from build123d import *


with BuildPart() as part:
    # Sketch1 → Base-Revolve (revolve)
    with BuildSketch(Plane.XY):
        with BuildLine():
            Line((132, 30), (0, 30))
            Line((0, 30), (-132, 30))
            Line((-132, 30), (-132, 28.5))
            Line((-132, 28.5), (-134.15, 28.5))
            Line((-134.15, 28.5), (-134.15, 30))
            Line((-134.15, 30), (-136.323673019, 30))
            ThreePointArc((-136.323673019, 30), (-136.497321197, 29.984807753), (-136.665693163, 29.939692621))
            Line((-136.665693163, 29.939692621), (-137.842020143, 29.511544614))
            ThreePointArc((-137.842020143, 29.511544614), (-138.319152044, 29.14542843), (-138.5, 28.571851993))
            Line((-138.5, 28.571851993), (-138.5, 0))
            Line((-138.5, 0), (115.555513627, 0))
            Line((115.555513627, 0), (118.5, 5.1))
            Line((118.5, 5.1), (138.5, 5.1))
            Line((138.5, 5.1), (138.5, 28.571851993))
            ThreePointArc((138.5, 28.571851993), (138.319152044, 29.14542843), (137.842020143, 29.511544614))
            Line((137.842020143, 29.511544614), (136.665693163, 29.939692621))
            ThreePointArc((136.665693163, 29.939692621), (136.497321197, 29.984807753), (136.323673019, 30))
            Line((136.323673019, 30), (134.15, 30))
            Line((134.15, 30), (134.15, 28.5))
            Line((134.15, 28.5), (132, 28.5))
            Line((132, 28.5), (132, 30))
        make_face()
    revolve(axis=Axis((-138.5, 0, 0), (1, 0, 0)))


solid = part.part
Design review of the part built by this model. Coordinates are the model's own, in mm. A direction names the side the tool comes from. Round coordinates to 2 decimals unless told otherwise and drop trailing zeros. Write each loop counter-clockwise with the first axis right and the second up, starting at its lowest first coordinate (ties: lowest second). Pieces come first, ordered by that corner, then holes. Notation, with made-up numbers: (46, -9) - (56, -9) arc R24 ccw to (56, 17) - close; hole circle Ø5 at (63, -29.75). An arc over 180 degrees is marked (long way). Use a Markdown table: item, result. Add a question column.
1. Mouldability with a two-part tool opening along Y and no side actions: class faces 3 (the face through (128.6, 2.4, -4.5)), 4 (the face through (134.15, 11, -27)), 5 (the face through (-133.09, 26.327, -10.916)) as +Y half, -Y half, draft (parallel to the pull), parting line (faces both ways), or undercut.
2. Wall thickness on probe 1 along Z at (x, y) = (124, 0); probe 2 along X at (y, z) = (27, 10.5); probe 3 along Z at (x, y) = (134, 0): over which ranges is each line inside the solid? List them lowest first.
3. For faces 1 (the face through (138.5, 0, -6)), 2 (the face through (-134.15, -11, -27)), list the 3-axis set-ups (+Z, -Z, +X, -X, +Y, -Y) from which the entire face can be reached by the end or side of a thin tool; tool diameter is ignored.
4. Clearance check with flat-ended pins moving along their axes: pin 1 (6 mm diameter, centred on x = -36.5, z = 12, fed in from -Y); pin 2 (8 mm diameter, centred on x = 82.5, y = -11.5, fed in from +Z); pin 3 (4 mm diameter, centred on x = -34.5, z = -18.5, fed in from +Y). State where each tip first meets the part, or that it passes through.
5. We need section A-A (x = -63.5). State the section outline as (y, z) points, then the cut area to 3 significant figures.
Output:
| question | item | result |
|---|---|---|
| 1 | face 3 | undercut |
| 1 | face 4 | draft |
| 1 | face 5 | parting line |
| 2 | probe 1 | z = -30 to -5.1, 5.1 to 30 |
| 2 | probe 2 | x = -138.42 to -134.15, -132 to 132, 134.15 to 138.42 |
| 2 | probe 3 | z = -28.5 to -5.1, 5.1 to 28.5 |
| 3 | face 1 | +Z, -Z, +X, +Y, -Y |
| 3 | face 2 | none |
| 4 | pin 1 | stops at y = -28.62 |
| 4 | pin 2 | stops at z = 29.05 |
| 4 | pin 3 | stops at y = 25.05 |
| 5 | outline | circle Ø60 at (0, 0) |
| 5 | area | 2,830 mm2 |
